Autodesk Inventor part; units mm, degrees
ref_plane "YZ Plane" through (0, 0, 0) normal (1, 0, 0) x (0, 1, 0)
ref_plane "XZ Plane" through (0, 0, 0) normal (0, 1, 0) x (-1, 0, 0)
ref_plane "XY Plane" through (0, 0, 0) normal (0, 0, 1) x (1, 0, 0)
sketch "Sketch1" plane through (0, 0, 0) normal (0, 0, 1) x (1, 0, 0)
  line L0 (-120, 0) -> (45, 0)
  circle A0 centre (0, -12.5) radius 4.05
  circle A1 centre (0, -87.5) radius 4.05
  line L1 (-120, 0) -> (-120, -5)
  line L2 (-120, -5) -> (-7.9396, -97.1546)
  arc A2 (-7.9396, -97.1546) -> (11.6724, -91.9728) centre (0, -87.5) ccw
  line L3 (11.6724, -91.9728) -> (45, -5)
  line L4 (45, -5) -> (45, 0)
  point P0 (0, 0)
  dimension "d0" = 12.5
  dimension "d1" = 75
  dimension "d2" = 8.1
  dimension "d3" = 165
  dimension "d4" = 12.5
  dimension "d5" = 5
  dimension "d6" = 45
extrude "Extrusion1" add sketch "Sketch1" along normal blind 5
sketch "Sketch2" plane through (0, 0, 5) normal (0, 0, 1) x (1, 0, 0)
  circle A0 centre (0, -87.5) radius 4.05
  circle A1 centre (0, -12.5) radius 4.05
  line L0 (45, 0) -> (-120, 0)
  line L1 (-120, 0) -> (-120, -5)
  arc A2 (-7.9396, -97.1546) -> (11.6724, -91.9728) centre (0, -87.5) ccw
  line L2 (45, -5) -> (45, 0)
  circle A3 centre (0, -87.5) radius 12.5
  line L3 (-120, -5) -> (-12.5, -5)
  line L4 (-12.5, -5) -> (-12.5, -87.5)
  line L5 (12.5, -87.5) -> (12.5, -5)
  line L6 (12.5, -5) -> (45, -5)
  point P0 (0, 0)
extrude "Extrusion2" add sketch "Sketch2" along normal blind 20
sketch "Sketch3" plane through (-120, -5, 5) normal (0, -1, 0) x (1, 0, 0)
  line L0 (107.5, 0) -> (0, 0)
  line L1 (0, 20) -> (107.5, 20)
  line L2 (0, 0) -> (0, 20)
  line L3 (165, 0) -> (132.5, 0)
  line L4 (165, 0) -> (165, 20)
  line L5 (132.5, 20) -> (165, 20)
  line L6 (132.5, 0) -> (132.5, 20)
  line L7 (7.5, 7.5) -> (157.5, 7.5)
  circle A0 centre (157.5, 7.5) radius 4.05
  circle A1 centre (7.5, 7.5) radius 4.05
  point P0 (120, -5)
  dimension "d11" = 8.1
  dimension "d13" = 150
  dimension "d14" = 7.5
  dimension "d15" = 12.5
extrude "Extrusion3" cut sketch "Sketch3" against normal through all contours A1 | A0
fillet "Fillet1" radius 5 2 edges at (12.5, -5, 15) (-12.5, -5, 15)
sketch "Sketch4" plane through (0, 0, 25) normal (0, 0, 1) x (1, 0, 0)
  circle A0 centre (0, -12.5) radius 4.05
  circle A1 centre (0, -87.5) radius 4.05
  arc A2 (-12.5, -87.5) -> (12.5, -87.5) centre (0, -87.5) ccw
  line L0 (7.5633, -12.5) -> (3.7816, -19.05)
  line L1 (3.7816, -19.05) -> (-3.7816, -19.05)
  line L2 (-3.7816, -19.05) -> (-7.5633, -12.5)
  line L3 (-7.5633, -12.5) -> (-3.7816, -5.95)
  line L4 (-3.7816, -5.95) -> (3.7816, -5.95)
  line L5 (3.7816, -5.95) -> (7.5633, -12.5)
  line L6 (7.5633, -87.5) -> (3.7816, -94.05)
  line L7 (3.7816, -94.05) -> (-3.7816, -94.05)
  line L8 (-3.7816, -94.05) -> (-7.5633, -87.5)
  line L9 (-7.5633, -87.5) -> (-3.7816, -80.95)
  line L10 (-3.7816, -80.95) -> (3.7816, -80.95)
  line L11 (3.7816, -80.95) -> (7.5633, -87.5)
  point P0 (0, 0)
  dimension "d19" = 13.1
extrude "Extrusion4" cut sketch "Sketch4" against normal blind 6
sketch "Sketch7" plane through (0, 0, 5) normal (0, 0, 1) x (1, 0, 0)
  line L0 (-120, -5) -> (-7.9396, -97.1546)
  circle A0 centre (-40.8613, -33.3613) radius 28.3613
  line L1 (-120, -5) -> (-17.5, -5)
  line L2 (-12.5, -10) -> (-12.5, -87.5)
  circle A1 centre (-40.8613, -33.3613) radius 20.8613
  point P0 (0, 0)
  dimension "d31" = 7.5
extrude "Extrusion7" cut sketch "Sketch7" against normal through all contours A1
sketch "Sketch8" plane through (0, 0, 5) normal (0, 0, 1) x (1, 0, 0)
  circle A0 centre (-40.8613, -33.3613) radius 20.8613
  line L0 (-120, -5) -> (-7.9396, -97.1546)
  circle A1 centre (-75.5091, -20.9444) radius 15.9444
  circle A2 centre (-75.5091, -20.9444) radius 8.4444
  line L1 (-120, -5) -> (-17.5, -5)
  point P0 (0, 0)
  dimension "d37" = 7.5
extrude "Extrusion8" cut sketch "Sketch8" against normal through all contours A2
sketch "Sketch9" plane through (0, 0, 5) normal (0, 0, 1) x (1, 0, 0)
  circle A0 centre (-40.8613, -33.3613) radius 20.8613
  line L0 (-120, -5) -> (-7.9396, -97.1546)
  circle A1 centre (-26.13, -64.5485) radius 13.63
  line L1 (-12.5, -10) -> (-12.5, -87.5)
  circle A2 centre (-26.13, -64.5485) radius 6.13
  point P0 (0, 0)
  dimension "d41" = 7.5
extrude "Extrusion9" cut sketch "Sketch9" against normal through all contours A2
sketch "Sketch10" plane through (0, 0, 5) normal (0, 0, 1) x (1, 0, 0)
  line L0 (11.6724, -91.9728) -> (45, -5)
  circle A0 centre (25.7431, -18.2431) radius 13.2431
  line L1 (17.5, -5) -> (45, -5)
  line L2 (12.5, -87.5) -> (12.5, -10)
  circle A1 centre (25.7431, -18.2431) radius 5.7431
  point P0 (0, 0)
  dimension "d45" = 7.5
extrude "Extrusion10" cut sketch "Sketch10" against normal through all contours A1
fillet "Fillet2" radius 7.5 2 edges at (-120, -2.5, 25) (45, -2.5, 25)
properties part number "board bracket right"
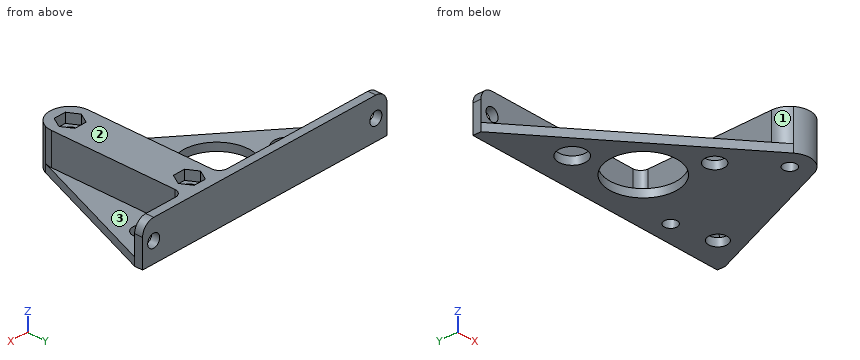
The listing builds one solid part. Answer for the finished solid, in the listing's coordinates (mm). Face numbers are marked on the shaded views. A direction names the side the tool comes from. Give positions to 0.01 mm unless a question says otherwise; leave off trailing zeros. Order: outer loops, then holes, each group sorted by start corner. A loop starts at its lowest first (then second) coordinate and runs counter-clockwise, first axis right, second up.
1) Find section C-C on x = -51.5. Write down the section's boundary in (y, z).
Reported:
outline: (-61.33, 0) - (-51.31, 0) - (-51.31, 5) - (-61.33, 5) - close; (-15.42, 0) - (0, 0) - (0, 25) - (-5, 25) - (-5, 5) - (-15.42, 5) - close
2) Consider line 1 along Y through (x, z) = (-39, 13.25); line 2 along Z through (x, y) = (-35, -8); line 3 along Z through (x, y) = (37.5, -1.9). Determine where each line is inside the solid, lowest interval first.
Reported:
line 1: y = -5 to 0
line 2: z = 0 to 5
line 3: z = 0 to 8.45, 16.55 to 25
3) Find section D-D on x = -26.13. Write down the section's boundary in (y, z).
Reported:
outline: (-82.2, 0) - (-70.68, 0) - (-70.68, 5) - (-82.2, 5) - close; (-58.42, 0) - (-48.13, 0) - (-48.13, 5) - (-58.42, 5) - close; (-18.59, 0) - (0, 0) - (0, 25) - (-5, 25) - (-5, 5) - (-18.59, 5) - close
4) For the marked faces 1, 2 and 3, determine the directions among +Z, -Z, +X, -X, +Y, -Y from which every point of the face is accessible in a straight line to the end or side of a thin tool.
Reported:
face 1: +Z, -X, -Y
face 2: +Z, +X, -X, +Y, -Y
face 3: +Z, +X, -Y
5) Find section A-A on z = 12.5. Write down the section's boundary in (x, y), then the cut area to 3 significant figures.
Reported:
outline: (-120, -5) - (-116.55, -5) - (-116.55, 0) - (-120, 0) - close; (-108.45, -5) - (-17.5, -5) arc R5 cw to (-12.5, -10) - (-12.5, -87.5) arc R12.5 ccw to (-7.94, -97.15) arc R12.5 ccw to (11.67, -91.97) arc R12.5 ccw to (12.5, -87.5) - (12.5, -10) arc R5 cw to (17.5, -5) - (33.45, -5) - (33.45, 0) - (-108.45, 0) - close; (41.55, -5) - (45, -5) - (45, 0) - (41.55, 0) - close; hole circle Ø8.1 at (0, -87.5); hole circle Ø8.1 at (0, -12.5)
area: 2,960 mm2
6) Find section B-B on x = 0. Write down the section's boundary in (y, z).
Reported:
outline: (-100, 0) - (-91.55, 0) - (-91.55, 19) - (-94.05, 19) - (-94.05, 25) - (-100, 25) - close; (-83.45, 0) - (-16.55, 0) - (-16.55, 19) - (-19.05, 19) - (-19.05, 25) - (-80.95, 25) - (-80.95, 19) - (-83.45, 19) - close; (-8.45, 0) - (0, 0) - (0, 25) - (-5.95, 25) - (-5.95, 19) - (-8.45, 19) - close
7) Given P1, Ø10, axis at x = 30.5, z = 14, coming from the -Y side; P2, Ø10, axis at y = -78, z = 11, coming from the -X side; P3, Ø10, axis at y = -53.5, z = 12, coming from the +X side, each flat-ended and moving along its own axis, determine where each tip first touches the part or whether it passes through.
Reported:
P1: stops at y = -5
P2: stops at x = -12.5
P3: stops at x = 12.5
